Model file for the job. Use its own axes, mm. Face numbers are marked on the shaded views. Round coordinates to 2 decimals unless told otherwise and drop trailing zeros. Loops run counter-clockwise (first coordinate to the right, second up) from the corner with the lowest first, then second, coordinate; pieces in that order, holes last. Notation, with made-up numbers: (47.5, 52) -> (69.5, 52) arc R13 ccw to (69.5, 75) -> close; hole circle Ø3 at (19.5, 62). An arc over 180 degrees is marked (long way). Use a Markdown table: item, result.
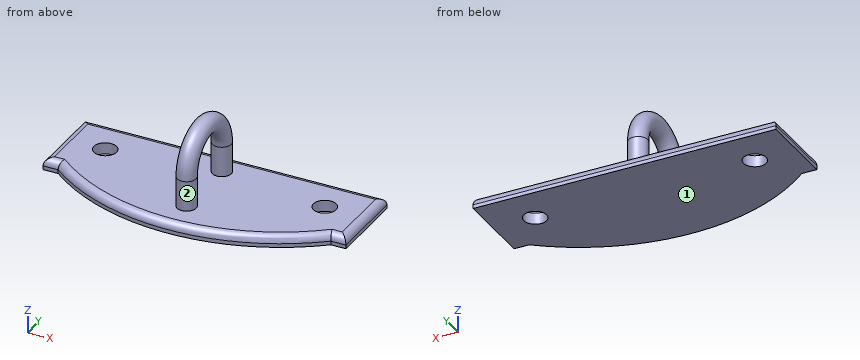
from build123d import *

# Parameters (mm, degrees)
BOSS_EXTRUDE1_DEPTH = 1.5
SKETCH2_R           = 1.5
CUT_EXTRUDE1_DEPTH  = 1.5
SKETCH3_R           = 1.25
FILLET1_R           = 1


with BuildPart() as part:
    # Sketch1 → Boss-Extrude1 (new body)
    with BuildSketch(Plane.XY):
        with BuildLine():
            Line((0, 0), (20, 0))
            Line((20, 0), (20, -10.5))
            Line((20, -10.5), (18, -10.5))
            ThreePointArc((18, -10.5), (0, -16.9094223), (-18, -10.5))
            Line((-18, -10.5), (-20, -10.5))
            Line((-20, -10.5), (-20, 0))
            Line((-20, 0), (0, 0))
        make_face()
    extrude(amount=BOSS_EXTRUDE1_DEPTH)

    # Sketch2 → Cut-Extrude1 (cut)
    with BuildSketch(Plane.XY.offset(1.5)):
        with Locations((-14.5, -5.25)):
            Circle(SKETCH2_R)
        with Locations((14.5, -5.25)):
            Circle(SKETCH2_R)
    extrude(amount=-CUT_EXTRUDE1_DEPTH, mode=Mode.SUBTRACT)

    # Sweep2: sweep along a path in Sketch4
    with BuildLine(Plane(origin=(0, 0, 0), x_dir=(0, 0, -1), z_dir=(1, 0, 0))) as sweep2_path:
        Line((-1.5, -3.5), (-5.5, -3.5))
        ThreePointArc((-5.5, -3.5), (-10, -8), (-5.5, -12.5))
        Line((-5.5, -12.5), (-1.5, -12.5))
    # Sketch3 → Sweep2 (sweep)
    with BuildSketch(Plane.XY.offset(1.5)):
        with Locations((0, -12.5)):
            Circle(SKETCH3_R)
    sweep(path=sweep2_path.line)

    # Fillet1
    fillet1_edges = [part.edges().sort_by_distance(p)[0] for p in [
        (-19, -10.5, 1.5),
        (0, -16.9094223, 1.5),
        (19, -10.5, 1.5),
        (20, -5.25, 1.5),
        (0, 0, 1.5),
        (-20, -5.25, 1.5),
    ]]
    fillet(fillet1_edges, radius=FILLET1_R)


solid = part.part
Q1. Drill centre lines: L1, parallel to Y at x = 0, z = 3.5; L2, parallel to Z at x = 2, y = -10.25; L3, parallel to Y at x = 14.5, z = 0.55. Where is each one in solid material? Low to high. Write a range as from..to.
Results list:
| item | result |
|---|---|
| L1 | y = -13.75..-11.25, -4.75..-2.25 |
| L2 | z = 0..1.5 |
| L3 | y = -12.94..-6.75, -3.75..0 |
Q2. Flat gauge pins, fed straight in: pin 1 (2 mm diameter, centred on x = -13.5, y = -6.5, fed in from +Z); pin 2 (0.6 mm diameter, centred on x = 19.5, z = 0, fed in from -Y). Where does each tip first touch, or does it go through?
Results list:
| item | result |
|---|---|
| pin 1 | stops at z = 1.5 |
| pin 2 | stops at y = -10.5 |
Q3. Band-saw the part on A-A, the plane x = 0. Give the cut face in (y, z).
Results list:
| item | result |
|---|---|
| outline | (-16.91, 0) -> (0, 0) -> (0, 0.5) arc R1 ccw to (-1, 1.5) -> (-2.25, 1.5) -> (-2.25, 5.5) arc R5.75 ccw to (-13.75, 5.5) -> (-13.75, 1.5) -> (-15.91, 1.5) arc R1 ccw to (-16.91, 0.5) -> close; hole (-11.25, 1.5) -> (-4.75, 1.5) -> (-4.75, 5.5) arc R3.25 ccw to (-11.25, 5.5) -> close |
Q4. Band-saw the part on B-B, the plane z = 3.5. Give the cut face in (x, y).
Results list:
| item | result |
|---|---|
| outline | circle Ø2.5 at (0, -12.5); circle Ø2.5 at (0, -3.5) |
Q5. Pull direction Y, two halves, no side cores. Call the marked faces 1 and 2: released by +Y, released by -Y, zero draft, split by the parting line, or undercut.
Results list:
| item | result |
|---|---|
| face 1 | zero draft |
| face 2 | undercut |
